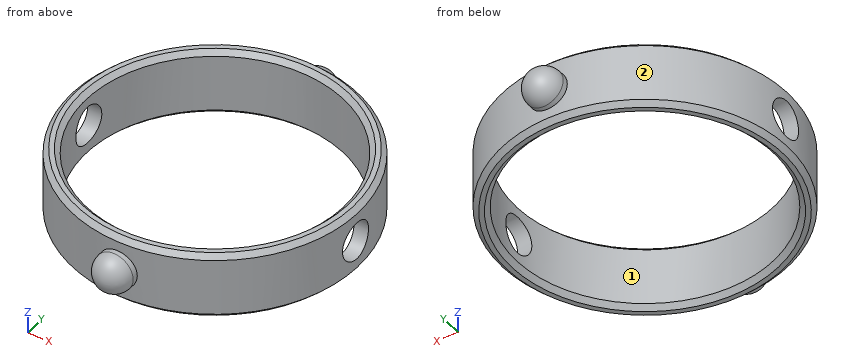
```python
from build123d import *

# Parameters (mm, degrees)
F0_R     = 15
F0_R_2   = 13.5
F1_DEPTH = 7
F2_R     = 2
F3_DEPTH = 20
F4_SIZE  = 0.5
F6_R     = 2
F7_DEPTH = 4
F9_R     = 2


with BuildPart() as f1:
    # F0 (on Top) → F1 (new body)
    with BuildSketch(Plane.XY):
        Circle(F0_R)
        Circle(F0_R_2, mode=Mode.SUBTRACT)
    extrude(amount=F1_DEPTH)

    # F2 (on Right) → F3 (cut, symmetric)
    with BuildSketch(Plane.YZ):
        with Locations((0, 3.5)):
            Circle(F2_R)
    extrude(amount=F3_DEPTH, both=True, mode=Mode.SUBTRACT)

    # F4
    f4_edges = [f1.edges().sort_by_distance(p)[0] for p in [
        (-15, 0, 7),
        (-13.5, 0, 7),
        (-15, 0, 0),
        (-13.5, 0, 0),
    ]]
    chamfer(f4_edges, length=F4_SIZE)

    # F6 (on offset) → F7 (join)
    with BuildSketch(Plane.XZ.offset(-13.5)):
        with Locations((0, 3.5)):
            Circle(F6_R)
    extrude(amount=-F7_DEPTH)

    # F8: F1 across plane


with BuildPart() as f1_1:
    add(f1.part)
    add(f1.part.mirror(Plane.XZ))

    # F9
    f9_edges = [f1_1.edges().sort_by_distance(p)[0] for p in [
        (-2, -17.5, 3.5),
        (-2, 17.5, 3.5),
    ]]
    fillet(f9_edges, radius=F9_R)


solid = f1_1.part
```
Here's how the part is built. I have some questions about the finished solid (model axes, mm). Face numbers are marked on the shaded views. Coordinates: 2 decimals unless noted, no trailing zeros. Write each loop counter-clockwise with the first axis right and the second up, starting at its lowest first coordinate (ties: lowest second). Pieces come first, ordered by that corner, then holes. Notation, with made-up numbers: M 3.5,-32.75 L 18.5,-32.75 A6 ccw 18.5,-27.75 Z; hole C 0,12.5 d7. An arc over 180 degrees is marked long. Answer as CSV lines item,"result". Start each with the question number.
Q1. Will these pins go through, and if not, where does the flat tip stop? pin 1 Ø2 at (x, y) = (-9.5, -9) entering from -Z; pin 2 Ø2.5 at (y, z) = (0, 3.5) entering from -X; pin 3 Ø1 at (y, z) = (-3.5, 1.5) entering from +X; pin 4 Ø4 at (y, z) = (9.5, 2) entering from -X.
Q2. Suppose I cut it at B-B, the plane y = 0. List the corners of the cut face in (x, z) for me, then the cut area to 3 significant figures.
Q3. Suppose I cut it at A-A, the plane x = 0. List the corners of the cut face in (y, z) for me, then the cut area to 3 significant figures.
Q4. I need wall thicknesses on probe 1 along X at (y, z) = (-3, 1); probe 2 along Y at (x, z) = (-13.7, 3.5); probe 3 along Y at (x, z) = (-0.5, 1.5). Which ranges of each line are inside material? Lowest first, please. Write a range as [from, to].
Q5. If we mould it in two halves opening along X, with no side actions, what happens to the marked faces 1 and 2? For each: pulls with the +X half, pulls with the -X half, needs draft (parallel to the pull), parting line crosses it, or undercut.
Q6. Suppose I cut it at C-C, the plane z = 3.5. List the corners of the cut face in (x, y) for me.
Entries:
1,pin 1,"stops at z = 0"
1,pin 2,"passes through"
1,pin 3,"stops at x = 14.7"
1,pin 4,"stops at x = -12.99"
2,outline,"M -15,0.5 L -14.5,0 L -14,0 L -13.5,0.5 L -13.5,1.5 L -15,1.5 Z; M -15,5.5 L -13.5,5.5 L -13.5,6.5 L -14,7 L -14.5,7 L -15,6.5 Z; M 13.5,0.5 L 14,0 L 14.5,0 L 15,0.5 L 15,1.5 L 13.5,1.5 Z; M 13.5,5.5 L 15,5.5 L 15,6.5 L 14.5,7 L 14,7 L 13.5,6.5 Z"
2,area,"8.00 mm²"
3,outline,"M -15.5,1.5 L -15,1.5 L -15,0.5 L -14.5,0 L -14,0 L -13.5,0.5 L -13.5,6.5 L -14,7 L -14.5,7 L -15,6.5 L -15,5.5 L -15.5,5.5 A2 ccw Z; M 13.5,0.5 L 14,0 L 14.5,0 L 15,0.5 L 15,1.5 L 15.5,1.5 A2 ccw 15.5,5.5 L 15,5.5 L 15,6.5 L 14.5,7 L 14,7 L 13.5,6.5 Z"
3,area,"36.6 mm²"
4,probe 1,"x = [-14.7, -13.16], [13.16, 14.7]"
4,probe 2,"y = [-6.11, -2], [2, 6.11]"
4,probe 3,"y = [-14.99, -13.49], [13.49, 14.99]"
5,face 1,"undercut"
5,face 2,"parting line crosses it"
6,outline,"M -14.87,-2 A15 ccw -2,-14.87 L -2,-15.5 A2 ccw 2,-15.5 L 2,-14.87 A15 ccw 14.87,-2 L 13.35,-2 A13.5 cw -13.35,-2 Z; M -14.87,2 L -13.35,2 A13.5 cw 13.35,2 L 14.87,2 A15 ccw 2,14.87 L 2,15.5 A2 ccw -2,15.5 L -2,14.87 A15 ccw Z"
